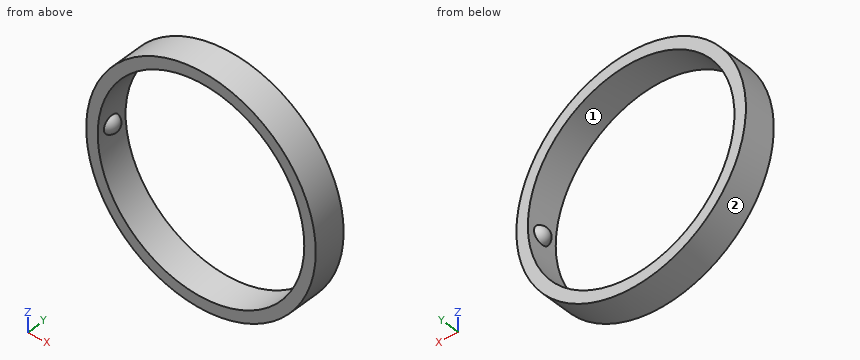
```python
from build123d import *

# Parameters (mm, degrees)
F0_R     = 25
F1_DEPTH = 7
F2_R     = 22.5
F3_DEPTH = 25


with BuildPart() as f1:
    # F0 (on Front) → F1 (new body)
    with BuildSketch(Plane.XZ):
        Circle(F0_R)
    extrude(amount=F1_DEPTH)

    # F2 (on face) → F3 (cut)
    with BuildSketch(Plane.XZ.offset(7)):
        Circle(F2_R)
    extrude(amount=-F3_DEPTH, mode=Mode.SUBTRACT)

    # F5 (on offset) → F6 (revolve)
    with BuildSketch(Plane.YZ.offset(23)):
        with BuildLine():
            Line((-5.5, 0), (-1.5, 0))
            ThreePointArc((-1.5, 0), (-3.5, 2), (-5.5, 0))
        make_face()
    revolve(axis=Axis((23, -3.548927, 0), (0, 1, 0)))

    # F7: F1 across plane


with BuildPart() as f1_1:
    add(f1.part)
    add(f1.part.mirror(Plane.YZ))


solid = f1_1.part
```
CAD build for the part. Positions are in the model's coordinates, mm. Face numbers are marked on the shaded views. Round coordinates to 2 decimals unless told otherwise and drop trailing zeros. Order: outer loops, then holes, each group sorted by start corner. A loop starts at its lowest first (then second) coordinate and runs counter-clockwise, first axis right, second up.
Item 1: Saw through at C-C on y = -2.75. Write the cut outline in (x, z).
Item 2: Probe line 1 along X through (y, z) = (-5.5, 0); line 2 along X through (y, z) = (-3, -19). List the from-to ranges inside material, lowest first.
Item 3: Mould opens along Z. For the marked faces 1 and 2 say: pulls with the +Z half, pulls with the -Z half, needs draft (parallel to the pull), parting line crosses it, or undercut.
Item 4: Saw through at B-B on z = 0. Write the cut outline in (x, y).
Item 5: Saw through at A-A on x = 0. Write the cut outline in (y, z), then the cut area to 3 significant figures.
Item 6: Saw through at D-D on z = 13.5. Write the cut outline in (x, y).
Item 7: Pin check, flat tips, straight feed: pin 1 (1.5 mm diameter, centred on y = -2, z = -7.5, fed in from -X); pin 2 (1.5 mm diameter, centred on y = -3, z = -18, fed in from +X); pin 3 (1 mm diameter, centred on x = 10, y = -6, fed in from +Z). Stop position of each tip, or through.
Reported:
1. outline: circle Ø50 at (0, 0); hole (-22.43, -1.76) arc R22.5 ccw to (22.43, -1.76) arc R1.85 cw to (22.43, 1.76) arc R22.5 ccw to (-22.43, 1.76) arc R1.85 cw to start
2. line 1: x = -25 to -22.5, 22.5 to 25
2. line 2: x = -16.25 to -12.05, 12.05 to 16.25
3. face 1: undercut
3. face 2: parting line crosses it
4. outline: (-25, -7) - (-22.5, -7) - (-22.5, -5.44) arc R2 ccw to (-22.5, -1.56) - (-22.5, 0) - (-25, 0) - close; (22.5, -7) - (25, -7) - (25, 0) - (22.5, 0) - (22.5, -1.56) arc R2 ccw to (22.5, -5.44) - close
5. outline: (-7, -25) - (0, -25) - (0, -22.5) - (-7, -22.5) - close; (-7, 22.5) - (0, 22.5) - (0, 25) - (-7, 25) - close
5. area: 35.0 mm2
6. outline: (-21.04, -7) - (-18, -7) - (-18, 0) - (-21.04, 0) - close; (18, -7) - (21.04, -7) - (21.04, 0) - (18, 0) - close
7. pin 1: stops at x = -24.07
7. pin 2: stops at x = 18.1
7. pin 3: stops at z = 23.12
